Build history of the part. All positions in model axes, mm. Face numbers are marked on the shaded views. A direction names the side the tool comes from. Round coordinates to 2 decimals unless told otherwise and drop trailing zeros. Loops run counter-clockwise (first coordinate to the right, second up) from the corner with the lowest first, then second, coordinate; pieces in that order, holes last. Notation, with made-up numbers: (-1.75, 23) - (39.25, 23) arc R33 cw to (39.25, 55) - close; hole circle Ø9 at (-10, -23). An arc over 180 degrees is marked (long way). Use one line per item in the form item = value. Start each with the question number.
Q1. Saw through at A-A (y = 240.5). Give the cut face in (x, z).
Q2. Saw through at C-C (z = 9). Give the cut face in (x, y).
Q3. Mould opens along Z. For the marked faces 1, 2, 3 and 4 say: released by +Z, released by -Z, zero draft, split by the parting line, or undercut.
Q4. Drill centre lines: line 1 (Y direction, x = -271, z = 7.2); line 2 (Y direction, x = -271, z = 5.2); line 3 (Z direction, x = -252, y = 258.5). Where is each one in solid material? Low to high.
Q5. 3-axis set-ups, long thin cutter, end or side, ignore diameter. For the marked faces 5, 6 and 7: which of +Z, -Z, +X, -X, +Y, -Y reach the whole face in a straight line?
Q6. Pin check, flat tips, straight feed: pin 1 (1.8 mm diameter, centred on x = -247.79, y = 271, fed in from -Z); pin 2 (5 mm diameter, centred on y = 248, z = 22, fed in from -X); pin 3 (11 mm diameter, centred on y = 241.5, z = 9.5, fed in from +X); pin 4 (2 mm diameter, centred on x = -266, z = 21.5, fed in from +Y). Stop position of each tip, or through.
Q7. Saw through at B-B (x = -248.5). Give the cut face in (y, z).
Q8. Saw through at D-D (x = -264). Give the cut face in (y, z).
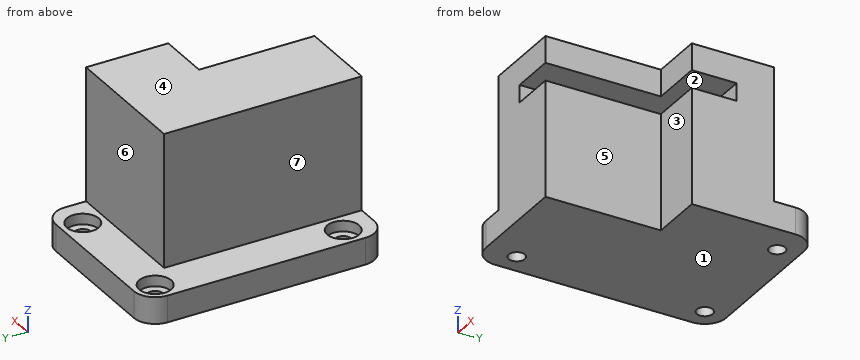
```python
from build123d import *

# Parameters (mm, degrees)
SKETCH021_W     = 33
SKETCH021_H     = 45
PAD004_DEPTH    = 30
POCKET012_DEPTH = 25
SKETCH023_R     = 1.5
POCKET013_DEPTH = 5.001
SKETCH024_R     = 3
POCKET014_DEPTH = 2
FILLET005_R     = 4
SKETCH025_W     = 22.162351
SKETCH025_H     = 3.3
POCKET015_DEPTH = 30
SKETCH026_W     = 15.81044
SKETCH026_H     = 25.49089
POCKET016_DEPTH = 30.001


with BuildPart() as part:
    # Sketch021 → Pad004 (new body)
    with BuildSketch(Plane.XY):
        with Locations((-258.5, 252.5)):
            Rectangle(SKETCH021_W, SKETCH021_H)
    extrude(amount=PAD004_DEPTH)

    # Sketch022 (on Face6 of Pad004) → Pocket012 (cut)
    with BuildSketch(Plane.XY.offset(30)):
        Polygon((-302.024292, 225.851654), (-267, 225.851654), (-267, 267), (-233.564453, 267), (-233.564453, 282.862976), (-302.024292, 282.862976), align=None)
    extrude(amount=-POCKET012_DEPTH, mode=Mode.SUBTRACT)

    # Sketch023 (on Face6 of Pocket012) → Pocket013 (cut, through all)
    with BuildSketch(Plane.XY.offset(5)):
        with Locations((-247.791107, 271)):
            Circle(SKETCH023_R)
        with Locations((-271, 235.791107)):
            Circle(SKETCH023_R)
        with Locations((-271, 271)):
            Circle(SKETCH023_R)
    extrude(amount=-POCKET013_DEPTH, mode=Mode.SUBTRACT)

    # Sketch024 (on Face6 of Pocket013) → Pocket014 (cut)
    with BuildSketch(Plane.XY.offset(5)):
        with Locations((-271, 271)):
            Circle(SKETCH024_R)
        with Locations((-247.791107, 271)):
            Circle(SKETCH024_R)
        with Locations((-271, 235.791107)):
            Circle(SKETCH024_R)
    extrude(amount=-POCKET014_DEPTH, mode=Mode.SUBTRACT)

    # Fillet005
    fillet005_edges = [part.edges().sort_by_distance(p)[0] for p in [
        (-275, 275, 2.5),
        (-242, 275, 2.5),
        (-275, 230, 2.5),
    ]]
    fillet(fillet005_edges, radius=FILLET005_R)

    # Sketch025 (on Face1 of Fillet005) → Pocket015 (cut)
    with BuildSketch(Plane.XZ.offset(-230)):
        with Locations((-249.108824, 23.35)):
            Rectangle(SKETCH025_W, SKETCH025_H)
    extrude(amount=-POCKET015_DEPTH, mode=Mode.SUBTRACT)

    # Sketch026 (on Face7 of Pocket015) → Pocket016 (cut, through all)
    with BuildSketch(Plane.XY.offset(30)):
        with Locations((-243.98507, 238.870476)):
            Rectangle(SKETCH026_W, SKETCH026_H)
    extrude(amount=-POCKET016_DEPTH, mode=Mode.SUBTRACT)


with BuildPart() as part_1:
    # Body004 placement: moved
    add(part.part.moved(Location((0, 0, 3))))


solid = part_1.part
```
Report:
q1.outline = (-275, 3) - (-251.89, 3) - (-251.89, 24.7) - (-260.19, 24.7) - (-260.19, 28) - (-251.89, 28) - (-251.89, 33) - (-267, 33) - (-267, 8) - (-275, 8) - close
q2.outline = (-267, 230) - (-251.89, 230) - (-251.89, 251.62) - (-242, 251.62) - (-242, 267) - (-267, 267) - close
q3.face_1 = released by -Z
q3.face_2 = undercut
q3.face_3 = zero draft
q3.face_4 = released by +Z
q4.line_1 = 230 to 232.79, 238.79 to 268, 274 to 275
q4.line_2 = 230 to 234.29, 237.29 to 269.5, 272.5 to 275
q4.line_3 = 3 to 24.7, 28 to 33
q5.face_5 = +Z, -Z, +X, -Y
q5.face_6 = +Z, +X, -X, +Y
q5.face_7 = +Z, -X, +Y, -Y
q6.pin_1 = through
q6.pin_2 = -267
q6.pin_3 = -251.89
q6.pin_4 = 267
q7.outline = (251.62, 3) - (269.68, 3) - (269.68, 6) - (268.08, 6) - (268.08, 8) - (267, 8) - (267, 33) - (251.62, 33) - (251.62, 28) - (260, 28) - (260, 24.7) - (251.62, 24.7) - close; (272.32, 3) - (275, 3) - (275, 8) - (273.92, 8) - (273.92, 6) - (272.32, 6) - close
q8.outline = (230, 3) - (275, 3) - (275, 8) - (267, 8) - (267, 33) - (230, 33) - close
